Here's the drawing with two shaded views (mm, measured from the low corner). I have some questions. A direction names the side the tool comes from. Give positions to 0.01 mm unless a question says otherwise; leave off trailing zeros. Write each loop counter-clockwise with the first axis right and the second up, starting at its lowest first coordinate (ties: lowest second). Pieces come first, ordered by that corner, then holes. Notation, with made-up numbers: (24.25, -18.5) -> (79.25, -18.5) arc R35 ccw to (79.25, 17.5) -> close; hole circle Ø1 at (77.5, 36.25). An arc over 180 degrees is marked (long way). One line per item, written item: value.
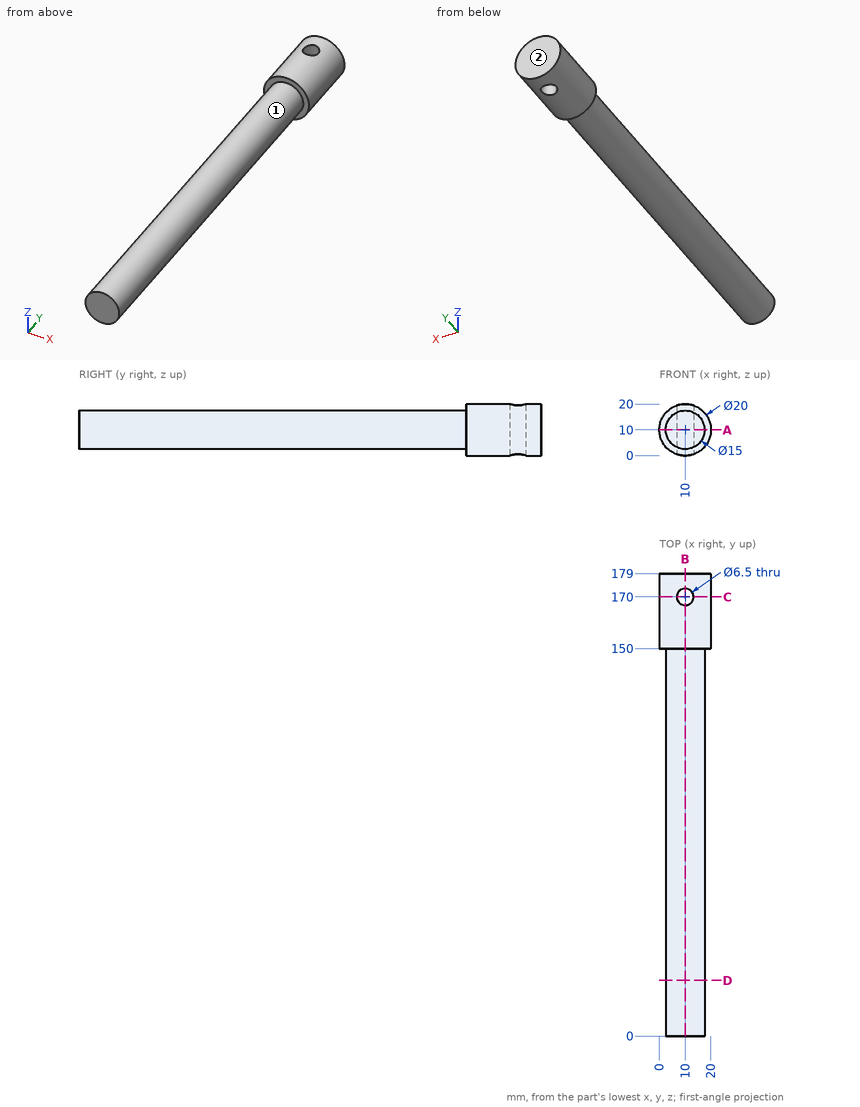
1) If we section it at D-D (y = 21.5): Write out the boundary of the cut face in (x, z), and give its area (3 significant figures).
Answer list:
outline: circle Ø15 at (10, 10)
area: 177 mm^2
2) If we section it at A-A (z = 10): Write out the boundary of the cut face in (x, y), and give its area (3 significant figures).
Answer list:
outline: (0, 150) -> (2.5, 150) -> (2.5, 0) -> (17.5, 0) -> (17.5, 150) -> (20, 150) -> (20, 179) -> (0, 179) -> close; hole circle Ø6.5 at (10, 170)
area: 2,800 mm^2
3) If we section it at C-C (y = 170): Write out the boundary of the cut face in (x, z), and give its area (3 significant figures).
Answer list:
outline: (6.75, 0.54) -> (6.75, 19.46) arc R10 ccw to start; (13.25, 0.54) arc R10 ccw to (13.25, 19.46) -> close
area: 186 mm^2
4) I need wall thicknesses on L1, parallel to X at y = 170, z = 10.5; L2, parallel to Y at x = 10.5, z = 5.5; L3, parallel to Y at x = 7.25, z = 1.5. Which ranges of each line are inside material? Lowest first, please.
Answer list:
L1: x = 0.01 to 6.75, 13.25 to 19.99
L2: y = 0 to 166.79, 173.21 to 179
L3: y = 150 to 168.27, 171.73 to 179
5) If we section it at B-B (x = 10): Write out the boundary of the cut face in (y, z).
Answer list:
outline: (0, 2.5) -> (150, 2.5) -> (150, 0) -> (166.75, 0) -> (166.75, 20) -> (150, 20) -> (150, 17.5) -> (0, 17.5) -> close; (173.25, 0) -> (179, 0) -> (179, 20) -> (173.25, 20) -> close
6) Will these pins go through, and if not, where does the flat tip stop? pin 1 (1 mm diameter, centred on x = 15.5, y = 102, fed in from +Z); pin 2 (8 mm diameter, centred on x = 9, y = 104.5, fed in from -Z); pin 3 (4 mm diameter, centred on y = 125, z = 7.5, fed in from +X); pin 4 (6 mm diameter, centred on x = 10, y = 170, fed in from -Z).
Answer list:
pin 1: stops at z = 15.59
pin 2: stops at z = 2.5
pin 3: stops at x = 17.48
pin 4: passes through
7) For the marked faces 1 and 2, which set-ups out of +Z, -Z, +X, -X, +Y, -Y let a thin tool reach every point of the face, with its end or its side?
Answer list:
face 1: -Y
face 2: +Z, -Z, +X, -X, +Y
